Autodesk Inventor part; units mm, degrees
ref_plane "dp1_XY" through (12.7, 7.9057, 0) normal (0, 0, 1) x (1, 0, 0)
ref_plane "dp1_YZ" through (12.7, 7.9057, 0) normal (1, 0, 0) x (0, 1, 0)
ref_plane "dp1_ZX" through (12.7, 7.9057, 0) normal (0, 1, 0) x (0, 0, 1)
sketch "Sketch_2" plane through (0, 0, 0) normal (0, 0, 1) x (1, 0, 0)
  line L0 (12.7, 0) -> (0, 0)
  line L1 (0, 0) -> (0, 7.098)
  line L2 (0, 7.098) -> (0.8395, 7.9375)
  line L3 (0.8395, 7.9375) -> (6.6726, 7.9375)
  line L4 (6.6726, 7.9375) -> (7.5126, 7.0988)
  arc A0 (7.5126, 7.0988) -> (8.1407, 6.839) centre (8.1407, 7.728) ccw
  line L5 (8.1407, 6.839) -> (9.4234, 6.839)
  arc A1 (9.4234, 6.839) -> (10.3124, 7.7279) centre (9.4234, 7.7279) ccw
  line L6 (10.3124, 7.7279) -> (10.3124, 7.9057)
  line L7 (10.3124, 7.9057) -> (12.7, 7.9057)
  line L8 (12.7, 7.9057) -> (12.7, 0)
  line L9 (12.7, 0) -> (0, 0)
revolve "Revolution1" add sketch "Sketch_2" angle 360 about axis through (12.7, 0, 0) along (1, 0, 0)
thread "Thread1"
sketch "Sketch_3" plane through (0, 0, 0) normal (0, 0, 1) x (1, 0, 0)
  line L0 (41.275, 0) -> (12.7, 0)
  line L1 (12.7, 0) -> (12.7, 13.3731)
  line L2 (12.7, 13.3731) -> (13.462, 14.1351)
  line L3 (13.462, 14.1351) -> (34.8615, 14.1351)
  line L4 (34.8615, 14.1351) -> (34.8615, 12.846)
  line L5 (34.8615, 12.846) -> (35.6235, 12.846)
  line L6 (35.6235, 12.846) -> (36.3855, 13.6081)
  line L7 (36.3855, 13.6081) -> (40.513, 13.6081)
  line L8 (40.513, 13.6081) -> (41.275, 12.846)
  line L9 (41.275, 12.846) -> (41.275, 0)
  line L10 (41.275, 0) -> (12.7, 0)
revolve "Revolution2" add sketch "Sketch_3" angle 360 about axis through (41.275, 0, 0) along (1, 0, 0)
sketch "Sketch3" plane through (0, 0, 0) normal (-1, 0, 0) x (0, 0, 1)
  point P0 (0, 0)
hole "Hole1" at (0, 0, 0) direction (1, 0, 0) diameter 8.0264 depth 41.275 countersink diameter 9.5504 countersink angle 90
sketch "Sketch_43" plane through (0, 0, 0) normal (0, 0, 1) x (1, 0, 0)
  line L0 (27.0002, 0) -> (27.0002, 14.1351)
  line L1 (27.0002, 14.1351) -> (32.4549, 14.1351)
  line L2 (32.4549, 14.1351) -> (31.8199, 13.5001)
  line L3 (31.8199, 13.5001) -> (31.5423, 4.6101)
  line L4 (31.5423, 4.6101) -> (30.1752, 3.8208)
  line L5 (30.1752, 3.8208) -> (30.1752, 0)
  line L6 (30.1752, 0) -> (27.0002, 0)
  line L7 (27.0002, 0) -> (27.0002, 14.1351)
revolve "Revolution3" cut sketch "Sketch_43" angle 360 about axis through (27.0002, 0, 0) along (0, -1, 0)
thread "Thread2"
sketch "Sketch_47" plane through (0, 0, 0) normal (0, 0, 1) x (1, 0, 0)
  line L0 (35.6235, 0) -> (34.8615, 0)
  line L1 (34.8615, 13.449) -> (34.8615, 12.5921)
  line L2 (34.8615, 12.5921) -> (35.6235, 12.5921)
  line L3 (35.6235, 12.5921) -> (35.6235, 12.846)
  line L4 (35.6235, 12.846) -> (35.2425, 12.846)
  line L5 (35.2425, 12.846) -> (34.984, 13.1046)
  arc A0 (34.984, 13.2842) -> (34.984, 13.1046) centre (35.0738, 13.1944) ccw
  line L6 (34.984, 13.2842) -> (35.7508, 14.0509)
  line L7 (35.7508, 14.0509) -> (35.7508, 14.1351)
  line L8 (35.7508, 14.1351) -> (35.5476, 14.1351)
  line L9 (35.5476, 14.1351) -> (34.8615, 13.449)
revolve "Revolution4" add sketch "Sketch_47" angle 360 about axis through (35.6235, 0, 0) along (1, 0, 0)
ref_plane "dp1_XY" through (12.7, 7.9057, 0) normal (0, 0, 1) x (1, 0, 0)
ref_plane "dp1_YZ" through (12.7, 7.9057, 0) normal (1, 0, 0) x (0, 1, 0)
ref_plane "dp1_ZX" through (12.7, 7.9057, 0) normal (0, 1, 0) x (0, 0, 1)
ref_plane "dp2_XY" through (12.7, -7.9057, 0) normal (0, 0, 1) x (1, 0, 0)
ref_plane "dp2_YZ" through (12.7, -7.9057, 0) normal (1, 0, 0) x (0, 1, 0)
ref_plane "dp2_ZX" through (12.7, -7.9057, 0) normal (0, 1, 0) x (0, 0, 1)
ref_plane "hh_XY" through (0, 7.9375, 0) normal (0, 0, 1) x (1, 0, 0)
ref_plane "hh_YZ" through (0, 7.9375, 0) normal (1, 0, 0) x (0, 1, 0)
ref_plane "hh_ZX" through (0, 7.9375, 0) normal (0, 1, 0) x (0, 0, 1)
ref_plane "port_XY" through (27.0002, 14.1351, 0) normal (0, 0, 1) x (1, 0, 0)
ref_plane "port_YZ" through (27.0002, 14.1351, 0) normal (1, 0, 0) x (0, 1, 0)
ref_plane "port_ZX" through (27.0002, 14.1351, 0) normal (0, 1, 0) x (0, 0, 1)
ref_plane "rod_guide_XY" through (0, 0, 0) normal (1, 0, 0) x (0, 0, -1)
ref_plane "rod_guide_YZ" through (0, 0, 0) normal (0, 0, -1) x (0, 1, 0)
ref_plane "rod_guide_ZX" through (0, 0, 0) normal (0, 1, 0) x (1, 0, 0)
ref_plane "s1_XY" through (10.3124, 0, 0) normal (0, 0, 1) x (1, 0, 0)
ref_plane "s1_YZ" through (10.3124, 0, 0) normal (1, 0, 0) x (0, 1, 0)
ref_plane "s1_ZX" through (10.3124, 0, 0) normal (0, 1, 0) x (0, 0, 1)
ref_plane "s2_XY" through (12.7, 0, 0) normal (0, 0, 1) x (1, 0, 0)
ref_plane "s2_YZ" through (12.7, 0, 0) normal (1, 0, 0) x (0, 1, 0)
ref_plane "s2_ZX" through (12.7, 0, 0) normal (0, 1, 0) x (0, 0, 1)
ref_plane "t1_XY" through (12.7, 0, 0) normal (1, 0, 0) x (0, 0, -1)
ref_plane "t1_YZ" through (12.7, 0, 0) normal (0, 0, -1) x (0, 1, 0)
ref_plane "t1_ZX" through (12.7, 0, 0) normal (0, 1, 0) x (1, 0, 0)
ref_plane "t111_XY" through (12.7, 0, 0) normal (1, 0, 0) x (0, 0, -1)
ref_plane "t111_YZ" through (12.7, 0, 0) normal (0, 0, -1) x (0, 1, 0)
ref_plane "t111_ZX" through (12.7, 0, 0) normal (0, 1, 0) x (1, 0, 0)
ref_plane "to_foot_bracket_XY" through (12.7, 0, 0) normal (1, 0, 0) x (0, 0, -1)
ref_plane "to_foot_bracket_YZ" through (12.7, 0, 0) normal (0, 0, -1) x (0, 1, 0)
ref_plane "to_foot_bracket_ZX" through (12.7, 0, 0) normal (0, 1, 0) x (1, 0, 0)
ref_plane "to_nut_XY" through (10.3124, 0, 0) normal (1, 0, 0) x (0, 0, -1)
ref_plane "to_nut_YZ" through (10.3124, 0, 0) normal (0, 0, -1) x (0, 1, 0)
ref_plane "to_nut_ZX" through (10.3124, 0, 0) normal (0, 1, 0) x (1, 0, 0)
ref_plane "to_rod_XY" through (0, 0, 0) normal (1, 0, 0) x (0, 0, -1)
ref_plane "to_rod_YZ" through (0, 0, 0) normal (0, 0, -1) x (0, 1, 0)
ref_plane "to_rod_ZX" through (0, 0, 0) normal (0, 1, 0) x (1, 0, 0)
ref_plane "to_screw_XY" through (27.0002, -7.0485, -10.2743) normal (0, 0, -1) x (1, 0, 0)
ref_plane "to_screw_YZ" through (27.0002, -7.0485, -10.2743) normal (1, 0, 0) x (0, -1, 0)
ref_plane "to_screw_ZX" through (27.0002, -7.0485, -10.2743) normal (0, -1, 0) x (0, 0, -1)
ref_plane "to_trunnion_brackets_XY" through (18.2118, 0, 0) normal (0, 1, 0) x (1, 0, 0)
ref_plane "to_trunnion_brackets_YZ" through (18.2118, 0, 0) normal (1, 0, 0) x (0, 0, -1)
ref_plane "to_trunnion_brackets_ZX" through (18.2118, 0, 0) normal (0, 0, -1) x (0, 1, 0)
ref_plane "to_trunnion_brackets1_XY" through (18.2118, 15.875, 0) normal (0, 1, 0) x (1, 0, 0)
ref_plane "to_trunnion_brackets1_YZ" through (18.2118, 15.875, 0) normal (1, 0, 0) x (0, 0, -1)
ref_plane "to_trunnion_brackets1_ZX" through (18.2118, 15.875, 0) normal (0, 0, -1) x (0, 1, 0)
ref_plane "to_trunnion_brackets2_XY" through (18.2118, -15.875, 0) normal (0, 1, 0) x (1, 0, 0)
ref_plane "to_trunnion_brackets2_YZ" through (18.2118, -15.875, 0) normal (1, 0, 0) x (0, 0, -1)
ref_plane "to_trunnion_brackets2_ZX" through (18.2118, -15.875, 0) normal (0, 0, -1) x (0, 1, 0)
ref_plane "to_tube_XY" through (35.6235, 0, 0) normal (1, 0, 0) x (0, 0, -1)
ref_plane "to_tube_YZ" through (35.6235, 0, 0) normal (0, 0, -1) x (0, 1, 0)
ref_plane "to_tube_ZX" through (35.6235, 0, 0) normal (0, 1, 0) x (1, 0, 0)
properties part number "09RK000-0_rod_guide"
Can you work these out from the model? Positions are in its coordinate system, mm. A direction names the side the tool comes from. Round coordinates to 2 decimals unless told otherwise and drop trailing zeros. Order: outer loops, then holes, each group sorted by start corner. A loop starts at its lowest first (then second) coordinate and runs counter-clockwise, first axis right, second up. Notation, with made-up numbers: (24.25, 47) -> (80.25, 47) arc R8 ccw to (80.25, 56) -> close; hole circle Ø11 at (-11.75, 75). An arc over 180 degrees is marked (long way). Write each question's results on one line, items separated by ' | '. Start each with the question number.
Item 1: Thinking about a two-plate mould opening in Z: for faces 4 (the cylindrical face through (24.31, -11.22, -8.6)), 5 (the flat face through (12.7, 6, -6)), 6 (the conical face through (31.93, 13.61, 0.07)), 7 (the conical face through (26.391, 9.117, -4.643)), which applies, +Z half, -Z half, draft (parallel to the pull), parting line (faces both ways), or undercut?
Item 2: Which directions (+Z, -Z, +X, -X, +Y, -Y) give clear straight access to the entire face, cutting with the end or side of a thin tool? Please do faces 1 (the cylindrical face through (3.8, -1.72, -7.75)), 2 (the conical face through (22.07, 13.61, -0.07)), 3 (the cylindrical face through (38.48, -10.8, -8.28)).
Item 3: If we section it at A-A, the plane x = 12: Write out the boundary of the cut face in (y, z).
Item 4: Please list where these lines run through material, in increasing order: L1, parallel to X at y = 8.25, z = -4 (3 decimals); L2, parallel to Z at x = 30.5, y = 0; L3, parallel to Z at x = 28.5, y = 1.75.
Item 5: Will these pins go through, and if not, where does the flat tip stop? pin 1 (6 mm diameter, centred on x = 6, y = -5.5, fed in from -Z); pin 2 (4.5 mm diameter, centred on y = 1.5, z = -4, fed in from -X); pin 3 (6.5 mm diameter, centred on y = 0, z = 0, fed in from +X); pin 4 (4 mm diameter, centred on x = 15, z = 11, fed in from -Y).
Item 6: If we section it at C-C, the plane x = 20.5: Write out the boundary of the cut face in (y, z), then the cut area to 3 significant figures.
Item 7: If we section it at B-B, the plane z = 0: State how many separate pieces and enclosed holes the cut face has, then the cut area to 3 significant figures.
Results:
1) face 4: parting line | face 5: draft | face 6: undercut | face 7: undercut
2) face 1: -X | face 2: +Y | face 3: +X
3) outline: circle Ø15.81 at (0, 0); hole circle Ø8.03 at (0, 0)
4) L1: x = 12.7 to 24.618, 29.383 to 41.275 | L2: z = -14.14 to -4.01, 4.01 to 14.14 | L3: z = -14.03 to -3.61, 3.61 to 14.03
5) pin 1: stops at z = -7.53 | pin 2: stops at x = 0 | pin 3: passes through | pin 4: stops at y = -10.9
6) outline: circle Ø28.27 at (0, 0); hole circle Ø8.03 at (0, 0) | area: 577 mm2
7) separate pieces: 3 | enclosed holes: 0 | area: 567 mm2
